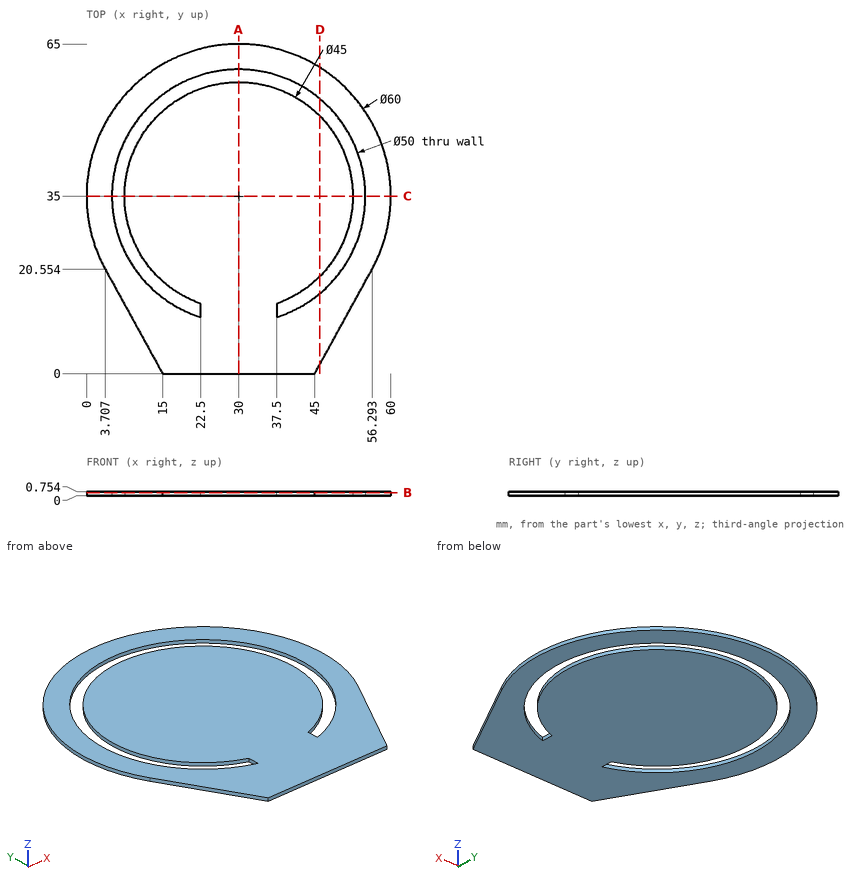
Can you work these out from the drawing? Everything is in mm from the part's minimum corner. Give positions to 0.01 mm unless a question says otherwise; leave off trailing zeros. Order: outer loops, then holes, each group sorted by start corner. A loop starts at its lowest first (then second) coordinate and runs counter-clockwise, first axis right, second up. Notation, with made-up numbers: M -37.5,45 L -3.5,45 A22 ccw -3.5,70 Z; hole C 51.5,21 d1. An arc over 180 degrees is marked long. One line per item, written item: value.
Item 1: If we section it at A-A on x = 30: Write out the boundary of the cut face in (y, z) (1 decimal).
Verdict:
outline: M 0,0 L 57.5,0 L 57.5,0.8 L 0,0.8 Z; M 60,0 L 65,0 L 65,0.8 L 60,0.8 Z
Item 2: Please list where these lines run through material, in increasing order: line 1 (X direction, y = 35, z = 0.5); line 2 (X direction, y = 24.5, z = 0.4); line 3 (Y direction, x = 9.5, z = 0.7) (1 decimal).
Verdict:
line 1: 0 to 5, 7.5 to 52.5, 55 to 60
line 2: 1.9 to 7.31, 10.1 to 49.9, 52.69 to 58.1
line 3: 10 to 20.7, 25.7 to 44.3, 49.3 to 56.9
Item 3: If we section it at C-C on y = 35: Write out the boundary of the cut face in (x, z) (1 decimal).
Verdict:
outline: M 0,0 L 5,0 L 5,0.8 L 0,0.8 Z; M 7.5,0 L 52.5,0 L 52.5,0.8 L 7.5,0.8 Z; M 55,0 L 60,0 L 60,0.8 L 55,0.8 Z
Item 4: If we section it at B-B on z = 0.55: Write out the boundary of the cut face in (x, y), and give its area (3 significant figures).
Verdict:
outline: M 3.71,20.55 L 15,0 L 45,0 L 56.29,20.55 A30 ccw long Z; hole M 22.5,11.15 L 22.5,13.79 A22.5 cw long 37.5,13.79 L 37.5,11.15 A25 ccw long Z
area: 2,760 mm2
Item 5: If we section it at D-D on x = 46: Write out the boundary of the cut face in (y, z) (1 decimal).
Verdict:
outline: M 1.8,0 L 15.8,0 L 15.8,0.8 L 1.8,0.8 Z; M 19.2,0 L 50.8,0 L 50.8,0.8 L 19.2,0.8 Z; M 54.2,0 L 60.4,0 L 60.4,0.8 L 54.2,0.8 Z
